Autodesk Inventor part; units mm, degrees
ref_plane "Work Plane1" through (2.9845, 0, 0) normal (1, 0, 0) x (0, 1, 0)
ref_plane "XZ Plane" through (0, 0, 0) normal (0, 1, 0) x (-1, 0, 0)
ref_plane "XY Plane" through (0, 0, 0) normal (0, 0, 1) x (1, 0, 0)
sketch "Sketch1" plane through (0, 0, 0) normal (0, 1, 0) x (-1, 0, 0)
  circle A0 centre (0, 0) radius 2.9845
  circle A1 centre (0, 0) radius 1.778
  dimension "d0" = 5.969
  dimension "d1" = 3.556
extrude "Extrusion1" add sketch "Sketch1" along normal blind 12.7
ref_plane "Work Plane1" through (2.9845, 0, 0) normal (1, 0, 0) x (0, 1, 0)
sketch "Sketch2" plane through (2.9845, 0, 0) normal (1, 0, 0) x (0, 1, 0)
  line L0 (6.35, 0) -> (0, 1.5875)
  line L1 (0, 1.5875) -> (0, -1.5875)
  line L2 (0, 2.9845) -> (0, -2.9845)
  line L3 (6.35, 0) -> (0, -1.5875)
  line L4 (0, -1.5875) -> (0, 0) construction
  line L5 (0, 0) -> (0, 1.5875) construction
  dimension "d4" = 3.175
  dimension "d5" = 6.35
extrude "Extrusion2" add sketch "Sketch2" along normal blind 0.635 and the other way blind 0.762
fillet "Fillet1" radius 0.254 1 edges at (3.302, 6.35, 0)
chamfer "Chamfer1" distance 4.572 distance2 0.381 1 edges at (3.6195, 0, 0) measured on face at (3.6195, 1.7881, 0.0821)
properties part number "HoleInsertsForBoltsLinkageSection" material "ABS Plastic"
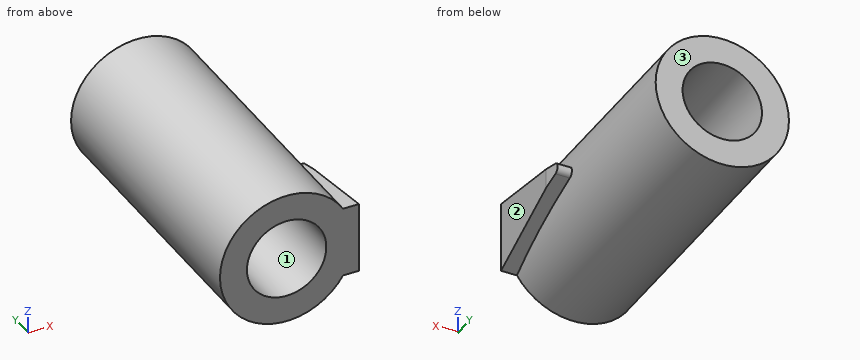
Source: CAD feature listing. Evaluate the final solid. Frame: model axes, mm. Face numbers are marked on the shaded views. Coordinates: 2 decimals unless noted, no trailing zeros. Order: outer loops, then holes, each group sorted by start corner. A loop starts at its lowest first (then second) coordinate and runs counter-clockwise, first axis right, second up.
Item 1: First-contact query: P1, Ø2, axis at x = 0.5, z = 1, coming from the -Y side. Flat tip, straight axial feed; report the tip coordinate or a pass-through.
Output values:
P1: stops at y = 0
Item 2: Cut plane B-B (z = 0). Return loops of the section in (x, y).
Output values:
outline: (-2.98, 0) - (-1.78, 0) - (-1.78, 12.7) - (-2.98, 12.7) - close; (1.78, 0) - (3.24, 0) - (3.62, 4.57) - (3.62, 5.56) - (2.98, 5.56) - (2.98, 12.7) - (1.78, 12.7) - close
Item 3: Cut plane A-A (x = 0). Return loops of the section in (y, z).
Output values:
outline: (0, -2.98) - (12.7, -2.98) - (12.7, -1.78) - (0, -1.78) - close; (0, 1.78) - (12.7, 1.78) - (12.7, 2.98) - (0, 2.98) - close
Item 4: Material intervals for line 1 (Z direction, x = 0, y = 8.25); line 2 (Z direction, x = -1.25, y = 7.75); line 3 (X direction, y = 1.25, z = -0.05), sorted ascending.
Output values:
line 1: z = -2.98 to -1.78, 1.78 to 2.98
line 2: z = -2.71 to -1.26, 1.26 to 2.71
line 3: x = -2.98 to -1.78, 1.78 to 3.34
Item 5: Cut plane D-D (x = -1). Return loops of the section in (y, z), plus the area to 3 significant figures.
Output values:
outline: (0, -2.81) - (12.7, -2.81) - (12.7, -1.47) - (0, -1.47) - close; (0, 1.47) - (12.7, 1.47) - (12.7, 2.81) - (0, 2.81) - close
area: 34.1 mm2
Item 6: Pull-direction query (X, two-part tool) for the marked faces 1, 2 and 3; classes: pulls with the +X half, pulls with the -X half, needs draft (parallel to the pull), parting line crosses it, or undercut.
Output values:
face 1: undercut
face 2: pulls with the +X half
face 3: needs draft
Item 7: Cut plane C-C (y = 3). Return loops of the section in (x, z).
Output values:
outline: (2.86, -0.84) - (3.49, -0.84) - (3.49, 0.84) - (2.86, 0.84) arc R2.98 ccw (long way) to start; hole circle Ø3.56 at (0, 0)
